Source: CAD feature listing. Evaluate the final solid. Frame: model axes, mm. A direction names the side the tool comes from. Give positions to 0.01 mm unless a question says otherwise; leave off trailing zeros. Write each loop counter-clockwise with the first axis right and the second up, starting at its lowest first coordinate (ties: lowest second). Pieces come first, ordered by that corner, then holes. Notation, with made-up numbers: (-33.5, 84) - (21.5, 84) arc R30 ccw to (21.5, 119) - close; hole circle Ø5 at (-26.5, 84). An arc over 180 degrees is marked (long way). Answer as a JSON object with one key per item and string values. Group by question number.
from build123d import *

# Parameters (mm, degrees)
F0_W     = 6.35
F0_H     = 12.7
F0_W_2   = 23.8125
F0_H_2   = 2.54
F0_H_3   = 0.76
F1_DEPTH = 26.825
F2_R     = 0.9525
F3_DEPTH = 18.541
F2_W     = 6.35
F2_H     = 6.35
F4_DEPTH = 3.81


with BuildPart() as f1:
    # F0 (on Top) → F1 (new body)
    with BuildSketch(Plane.XY):
        with Locations((-15.08125, 0)):
            Rectangle(F0_W, F0_H)
        Rectangle(F0_W_2, F0_H)
        with Locations((15.08125, 0)):
            Rectangle(F0_W, F0_H)
        with Locations((-15.08125, -7.62)):
            Rectangle(F0_W, F0_H_2)
        with Locations((-15.08125, -9.27)):
            Rectangle(F0_W, F0_H_3)
        Polygon((18.25625, -9.65), (11.90625, -9.65), (-11.90625, -9.65), (-18.25625, -9.65), (-18.25625, -12.19), (18.25625, -12.19), align=None)
        with Locations((0, -7.62)):
            Rectangle(F0_W_2, F0_H_2)
        with Locations((0, -9.27)):
            Rectangle(F0_W_2, F0_H_3)
        with Locations((15.08125, -7.62)):
            Rectangle(F0_W, F0_H_2)
        with Locations((15.08125, -9.27)):
            Rectangle(F0_W, F0_H_3)
    extrude(amount=F1_DEPTH)

    # F2 (on face) → F3 (cut, through all)
    with BuildSketch(Plane.XZ.offset(12.19)):
        Polygon((11.90625, 21.11), (11.90625, 24.285), (8.09625, 24.285), (-8.09625, 24.285), (-11.90625, 24.285), (-11.90625, 11.585), (11.90625, 11.585), (11.90625, 14.76), align=None)
        with Locations((-14.44625, 17.935)):
            Circle(F2_R)
        with Locations((14.44625, 17.935)):
            Circle(F2_R)
    extrude(amount=-F3_DEPTH, mode=Mode.SUBTRACT)

    # F2 (on face) → F4 (cut)
    with BuildSketch(Plane.XZ.offset(12.19)):
        with Locations((15.08125, 17.935)):
            Rectangle(F2_W, F2_H)
        with Locations((14.44625, 17.935)):
            Circle(F2_R, mode=Mode.SUBTRACT)
    extrude(amount=-F4_DEPTH, mode=Mode.SUBTRACT)


solid = f1.part
Q1. First-contact query: pin 1 Ø4 at (x, y) = (15, -10) entering from -Z; pin 2 Ø3 at (x, z) = (14.5, 18) entering from -Y. Flat tips, straight axial feed; report the tip coordinate or a pass-through.
Q2. Ray query, probe 1 along X at (y, z) = (3.5, 23.75); probe 2 along X at (y, z) = (-9.5, 18); probe 3 along Z at (x, y) = (0.5, -10.25) (3 decimals). Return the intervals inside material, ascending. Write a range as [from, to].
Q3. Draft query along X for faces 1 (the flat face through (0, -3, 0)), 2 (the cylindrical face through (14.24, -1.118, 17.005)), 3 (the flat face through (-18.256, -3, 13)), 4 (the flat face through (-11.906, -3, 18)). Return one class per face: released by +X, released by -X, zero draft, split by the parting line, or undercut.
Q4. Section C-C on y = -9.75. Return the cut outline in (x, z) (1 decimal).
Q5. Section B-B on z = 13.75. Return the cut outline in (x, y), then the cut area to 3 significant figures.
Q6. Section A-A on x = -1. Return the cut outline in (y, z) (3 decimals), then the cut area to 3 significant figures.
Q7. Reachability of faces 5 (the flat face through (11.906, -3, 18)), 6 (the flat face through (15, -10, 21.11)), 7 (the flat face through (0, -3, 26.825)) from +Z, -Z, +X, -X, +Y, -Y: full face, straight path, thin tool, end or side. Return the list, or none.
Q8. Section D-D on x = 13. Return the cut outline in (y, z) (3 decimals), then the cut area to 3 significant figures.
Taken from the geometry:
{
 "1": {"pin 1": "stops at z = 0", "pin 2": "stops at y = -8.38"},
 "2": {"probe 1": "x = [-18.26, -11.91], [11.91, 18.26]", "probe 2": "x = [-18.26, -15.4], [-13.5, -11.91]", "probe 3": "z = [0, 11.585], [24.285, 26.825]"},
 "3": {"face 1": "zero draft", "face 2": "undercut", "face 3": "released by -X", "face 4": "undercut"},
 "4": {"outline": "(-18.3, 0) - (18.3, 0) - (18.3, 14.8) - (11.9, 14.8) - (11.9, 11.6) - (-11.9, 11.6) - (-11.9, 24.3) - (11.9, 24.3) - (11.9, 21.1) - (18.3, 21.1) - (18.3, 26.8) - (-18.3, 26.8) - close; hole circle Ø1.9 at (-14.4, 17.9)"},
 "5": {"outline": "(-18.26, -12.19) - (-11.91, -12.19) - (-11.91, 6.35) - (-18.26, 6.35) - close; (11.91, -12.19) - (18.26, -12.19) - (18.26, 6.35) - (11.91, 6.35) - close", "area": "235 mm²"},
 "6": {"outline": "(-12.19, 0) - (6.35, 0) - (6.35, 11.585) - (-12.19, 11.585) - close; (-12.19, 24.285) - (6.35, 24.285) - (6.35, 26.825) - (-12.19, 26.825) - close", "area": "262 mm²"},
 "7": {"face 5": "+Y, -Y", "face 6": "+X, -Y", "face 7": "+Z, +X, -X, +Y, -Y"},
 "8": {"outline": "(-12.19, 0) - (6.35, 0) - (6.35, 26.825) - (-12.19, 26.825) - (-12.19, 21.11) - (-8.38, 21.11) - (-8.38, 14.76) - (-12.19, 14.76) - close", "area": "473 mm²"}
}
